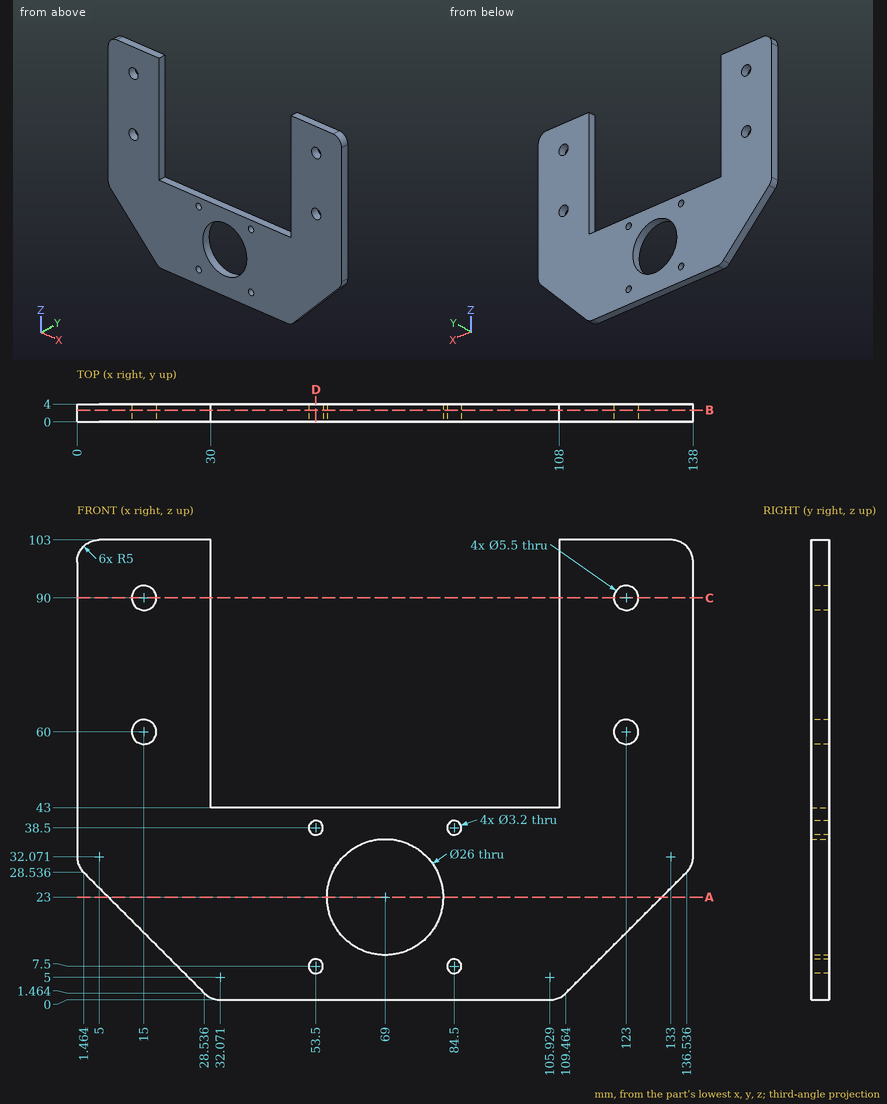
Here's the drawing with two shaded views (mm, measured from the low corner). I have some questions. Give positions to 0.01 mm unless a question says otherwise; leave off trailing zeros. Loops run counter-clockwise (first coordinate to the right, second up) from the corner with the lowest first, then second, coordinate; pieces in that order, holes last. Notation, with made-up numbers: M 12,14.5 L 53,14.5 A24 ccw 53,47.5 Z; hole C 52.25,0.5 d5. An arc over 180 degrees is marked long. One line per item, written item: value. Start each with the question number.
1) If we section it at A-A, the plane z = 23: Write out the boundary of the cut face in (x, y), and give its area (3 significant figures).
2) If we section it at B-B, the plane y = 2.6: Give the number of separate pieces and of enclosed holes in the cut face, and give its area (3 significant figures).
3) If we section it at D-D, the plane x = 53.5: Write out the boundary of the cut face in (y, z), and give its area (3 significant figures).
4) If I drill on line 1 (X direction, y = 1.55, z = 38.5); line 2 (Z direction, x = 53.5, y = 2.05); line 3 (X direction, y = 3, z = 90), over which ranges is the centre line in solid material (lowest first)? Write a range as [from, to].
5) I'm going to push flat-ended pins straight in: pin 1 (2.5 mm diameter, centred on x = 84.5, z = 38.5, fed in from -Y); pin 2 (1 mm diameter, centred on x = 52.5, y = 2.5, fed in from +Z). Where does each tip first touch, or does it pass through?
6) If we section it at C-C, the plane z = 90: Write out the boundary of the cut face in (x, y), and give its area (3 significant figures).
Completed:
1. outline: M 7,0 L 56,0 L 56,4 L 7,4 Z; M 82,0 L 131,0 L 131,4 L 82,4 Z
1. area: 392 mm^2
2. separate pieces: 1
2. enclosed holes: 9
2. area: 7,960 mm^2
3. outline: M 0,0 L 4,0 L 4,5.9 L 0,5.9 Z; M 0,9.1 L 4,9.1 L 4,36.9 L 0,36.9 Z; M 0,40.1 L 4,40.1 L 4,43 L 0,43 Z
3. area: 146 mm^2
4. line 1: x = [0, 51.9], [55.1, 82.9], [86.1, 138]
4. line 2: z = [0, 5.9], [9.1, 36.9], [40.1, 43]
4. line 3: x = [0, 12.25], [17.75, 30], [108, 120.25], [125.75, 138]
5. pin 1: passes through
5. pin 2: stops at z = 43
6. outline: M 0,0 L 12.25,0 L 12.25,4 L 0,4 Z; M 17.75,0 L 30,0 L 30,4 L 17.75,4 Z; M 108,0 L 120.25,0 L 120.25,4 L 108,4 Z; M 125.75,0 L 138,0 L 138,4 L 125.75,4 Z
6. area: 196 mm^2
